The drawing under review shows one solid part. Ordinate dimensions are in mm from its lowest x, y, z. Coordinates: 2 decimals unless noted, no trailing zeros. Write each loop counter-clockwise with the first axis right and the second up, starting at its lowest first coordinate (ties: lowest second). Pieces come first, ordered by that corner, then holes.
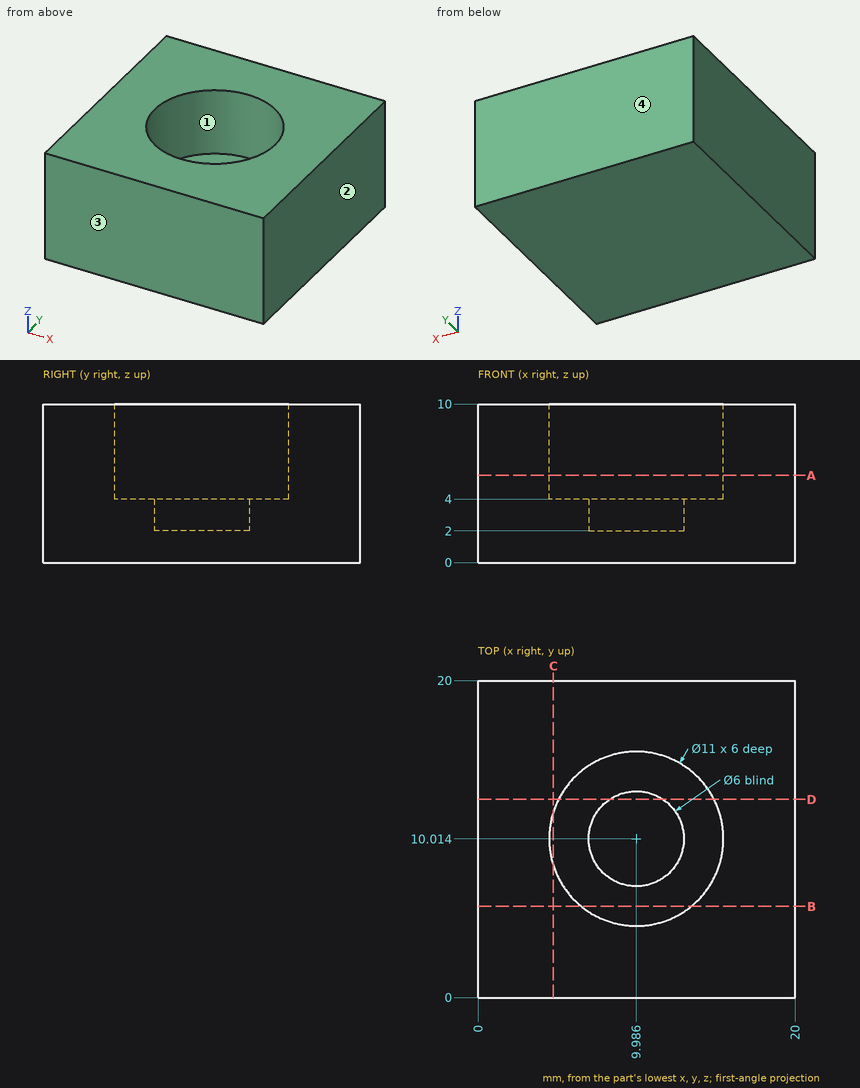
Q1. Add section B-B (y = 5.75). State the section outline as (x, z) points, then the cut area to 3 significant figures.
Ans:
outline: (0, 0) - (20, 0) - (20, 10) - (13.46, 10) - (13.46, 4) - (6.51, 4) - (6.51, 10) - (0, 10) - close
area: 158 mm2
Q2. Add section A-A (z = 5.5). State the section outline as (x, y) points (1 decimal), then the cut area to 3 significant figures.
Ans:
outline: (0, 0) - (20, 0) - (20, 20) - (0, 20) - close; hole circle Ø11 at (10, 10)
area: 305 mm2
Q3. Clearance check with flat-ended pins moving along their axes: pin 1 Ø1.8 at (x, y) = (10, 10) entering from +Z; pin 2 Ø9.5 at (x, y) = (9.99, 10.01) entering from +Z. State where each tip first meets the part, or that it passes through.
Ans:
pin 1: stops at z = 2
pin 2: stops at z = 4
Q4. Draft analysis for pull direction Y (two halves, no side actions). For the marked faces 1, 2, 3 and 4, state which applies: +Y half, -Y half, draft (parallel to the pull), parting line (faces both ways), or undercut.
Ans:
face 1: undercut
face 2: draft
face 3: -Y half
face 4: +Y half
Q5. Add section C-C (x = 4.75). State the section outline as (y, z) points.
Ans:
outline: (0, 0) - (20, 0) - (20, 10) - (11.7, 10) - (11.7, 4) - (8.33, 4) - (8.33, 10) - (0, 10) - close
Q6. For probe 1 along Z at (x, y) = (12.25, 11.5); probe 2 along Z at (x, y) = (6.25, 8); probe 3 along X at (y, z) = (14, 5) (1 decimal), list the stretches that pass through material, from the lowest coordinate up.
Ans:
probe 1: z = 0 to 2
probe 2: z = 0 to 4
probe 3: x = 0 to 6.2, 13.8 to 20
Q7. Add section D-D (y = 12.5). State the section outline as (x, z) points.
Ans:
outline: (0, 0) - (20, 0) - (20, 10) - (14.89, 10) - (14.89, 4) - (11.67, 4) - (11.67, 2) - (8.31, 2) - (8.31, 4) - (5.08, 4) - (5.08, 10) - (0, 10) - close
